Geometry check sheet. Reference: the model listing, model coordinates, mm. A direction names the side the tool comes from. Give positions to 0.01 mm unless a question says otherwise; leave off trailing zeros. Write each loop counter-clockwise with the first axis right and the second up, starting at its lowest first coordinate (ties: lowest second). Pieces come first, ordered by that corner, then holes. Notation, with made-up numbers: M 1.5,14.5 L 5.5,14.5 A23 cw 5.5,43.5 Z; hole C 74,-23 d3. An arc over 180 degrees is marked long. One line per item, written item: value. Start each with the question number.
1. Cross-section at D-D on x = 108.5. Record the cut outline in (y, z).
2. Tool access check on faces 4 (the face through (195.423, -46.748, 39.408)), 5 (the face through (43.2, -23.3, 33.5)), 6 (the face through (196, -47, 37.592)). Record the directions out of +Z, -Z, +X, -X, +Y, -Y that give a thin tool (end or side, any length) a straight path to the whole face; none if there is none.
3. Cross-section at B-B on z = 10. Count the separate pieces of the cut face and the enclosed holes in it, then the cut area to 3 significant figures.
4. Cross-section at C-C on y = -97. Record the cut outline in (x, z) (1 decimal).
5. Gauge pin test, flat ends, axial feed: pin 1 (0.8 mm diameter, centred on y = -98, z = 41, fed in from -X); pin 2 (9.5 mm diameter, centred on x = 62.23, y = -24.13, fed in from -Z); pin 3 (0.8 mm diameter, centred on y = -107.5, z = 41, fed in from +X). Record the tip position at first contact, or that the pin passes through.
6. Release check for a two-part mould opening along Y. For faces 1 (the face through (219.8, -6.44, 19.97)), 2 (the face through (195.423, -110.248, 39.408)), 3 (the face through (111, -74, 0)) record: pulls with the +Y half, pulls with the -Y half, needs draft (parallel to the pull), parting line crosses it, or undercut.
7. Scan lines: line 1 (Y direction, x = 30, z = 19); line 2 (X direction, y = -23, z = 19); line 3 (Y direction, x = 30.48, z = 19.5). Record each from-to range of solid material in increasing order.
8. Cross-section at A-A on x = 163.83. Record the cut outline in (y, z), then the cut area to 3 significant figures.
from build123d import *

# Parameters (mm, degrees)
SKETCH3_W                                        = 226.06
SKETCH3_H                                        = 149.86
EXTRUDE2_DEPTH                                   = 41.275
SKETCH4_W                                        = 226.06
SKETCH4_H                                        = 149.86
SKETCH4_W_2                                      = 22.225
SKETCH4_H_2                                      = 50.8
EXTRUDE4_DEPTH                                   = 0.762
CBORE_FOR_1_4_SOCKET_HEAD_CAP_SCREW1_AT_COUNT    = 2
CBORE_FOR_1_4_SOCKET_HEAD_CAP_SCREW1_AT_PITCH    = 186.028991356
CBORE_FOR_1_4_SOCKET_HEAD_CAP_SCREW1_2_COUNT     = 2
CBORE_FOR_1_4_SOCKET_HEAD_CAP_SCREW1_2_PITCH     = 166.589197204
CBORE_FOR_1_4_SOCKET_HEAD_CAP_SCREW1_3_COUNT     = 2
CBORE_FOR_1_4_SOCKET_HEAD_CAP_SCREW1_3_PITCH     = 63.5
F_1_4_20_TAPPED_HOLE1_D                          = 5.1054
CBORE_FOR_3_8_SOCKET_HEAD_CAP_SCREW1_D           = 10.31748
CBORE_FOR_3_8_SOCKET_HEAD_CAP_SCREW1_CBORE_D     = 38.1
CBORE_FOR_3_8_SOCKET_HEAD_CAP_SCREW1_CBORE_DEPTH = 14.224
SKETCH18_W                                       = 3.175
SKETCH18_H                                       = 133.35
CUT_EXTRUDE1_DEPTH                               = 0.762
F_10_32_TAPPED_HOLE1_D                           = 4.0386
CHAMFER1_SIZE                                    = 12.7


with BuildPart() as part:
    # Sketch3 → Extrude2 (new body)
    with BuildSketch(Plane.XY):
        with Locations((113.03, -74.93)):
            Rectangle(SKETCH3_W, SKETCH3_H)
    extrude(amount=EXTRUDE2_DEPTH)

    # Sketch4 → Extrude4 (cut)
    with BuildSketch(Plane.XY.offset(41.275)):
        with Locations((113.03, -74.93)):
            Rectangle(SKETCH4_W, SKETCH4_H)
        with Locations((30.4927, -33.655)):
            Rectangle(SKETCH4_W_2, SKETCH4_H_2, mode=Mode.SUBTRACT)
        with Locations((195.5673, -33.655)):
            Rectangle(SKETCH4_W_2, SKETCH4_H_2, mode=Mode.SUBTRACT)
        with Locations((30.4927, -116.205)):
            Rectangle(SKETCH4_W_2, SKETCH4_H_2, mode=Mode.SUBTRACT)
        with Locations((195.5673, -116.205)):
            Rectangle(SKETCH4_W_2, SKETCH4_H_2, mode=Mode.SUBTRACT)
    extrude(amount=-EXTRUDE4_DEPTH, mode=Mode.SUBTRACT)

    # Sketch9 → CBORE for 1/4 Socket Head Cap Screw1 (revolve, cut)
    with BuildSketch(Plane(origin=(195.58, -106.68, 0), x_dir=(0, 1, 0), z_dir=(1, 0, 0))):
        Polygon((0, 0), (0, 41.275), (3.57124, 41.275), (3.57124, 37.592), (5.55625, 37.592), (5.55625, 0.635), (6.19125, 0), align=None)
    cbore_for_1_4_socket_head_cap_screw1 = revolve(axis=Axis((195.58, -106.68, -6.35), (0, 0, 1)), mode=Mode.SUBTRACT)

    # CBORE for 1/4 Socket Head Cap Screw1 at: CBORE for 1/4 Socket Head Cap Screw1 ×2
    with Locations(*[Vector(-0.887496077, 0.460815271, 0) * (i * CBORE_FOR_1_4_SOCKET_HEAD_CAP_SCREW1_AT_PITCH) for i in range(1, CBORE_FOR_1_4_SOCKET_HEAD_CAP_SCREW1_AT_COUNT)]):
        add(cbore_for_1_4_socket_head_cap_screw1, mode=Mode.SUBTRACT)

    # CBORE for 1_4 Socket Head Cap Screw1 2: CBORE for 1/4 Socket Head Cap Screw1 ×2
    with Locations(*[Vector(-0.991060662, -0.133412012, 0) * (i * CBORE_FOR_1_4_SOCKET_HEAD_CAP_SCREW1_2_PITCH) for i in range(1, CBORE_FOR_1_4_SOCKET_HEAD_CAP_SCREW1_2_COUNT)]):
        add(cbore_for_1_4_socket_head_cap_screw1, mode=Mode.SUBTRACT)

    # CBORE for 1_4 Socket Head Cap Screw1 3: CBORE for 1/4 Socket Head Cap Screw1 ×2
    with Locations(*[(0, i * CBORE_FOR_1_4_SOCKET_HEAD_CAP_SCREW1_3_PITCH, 0) for i in range(1, CBORE_FOR_1_4_SOCKET_HEAD_CAP_SCREW1_3_COUNT)]):
        add(cbore_for_1_4_socket_head_cap_screw1, mode=Mode.SUBTRACT)

    # 1/4-20 Tapped Hole1 (through all)
    with Locations(Plane(origin=(0, 0, 0), x_dir=(-1, 0, 0), z_dir=(0, 0, -1))):
        with Locations((-195.58, -20.955), (-195.58, -128.905), (-30.48, -43.18), (-30.48, -106.68)):
            Hole(F_1_4_20_TAPPED_HOLE1_D / 2)

    # CBORE for 3/8 Socket Head Cap Screw1 (through all)
    with Locations(Plane.XY.offset(40.513)):
        with Locations((163.83, -125.73), (62.23, -125.73), (163.83, -24.13), (62.23, -24.13)):
            CounterBoreHole(CBORE_FOR_3_8_SOCKET_HEAD_CAP_SCREW1_D / 2, CBORE_FOR_3_8_SOCKET_HEAD_CAP_SCREW1_CBORE_D / 2, CBORE_FOR_3_8_SOCKET_HEAD_CAP_SCREW1_CBORE_DEPTH)

    # Sketch18 → Cut-Extrude1 (cut)
    with BuildSketch(Plane.XY.offset(41.275)):
        with Locations((30.48, -74.93)):
            Rectangle(SKETCH18_W, SKETCH18_H)
        with Locations((195.58, -74.93)):
            Rectangle(SKETCH18_W, SKETCH18_H)
    extrude(amount=-CUT_EXTRUDE1_DEPTH, mode=Mode.SUBTRACT)

    # #10-32 Tapped Hole1 (through all)
    with Locations(Plane(origin=(0, 0, 0), x_dir=(-1, 0, 0), z_dir=(0, 0, -1))):
        with Locations((-113.03, -13.0048), (-100.33, -136.8552), (-125.73, -136.8552)):
            Hole(F_10_32_TAPPED_HOLE1_D / 2)

    # Chamfer1
    chamfer1_edges = [part.edges().sort_by_distance(p)[0] for p in [
        (0, 0, 20.2565),
        (226.06, 0, 20.2565),
        (226.06, -149.86, 20.2565),
        (0, -149.86, 20.2565),
    ]]
    chamfer(chamfer1_edges, length=CHAMFER1_SIZE)


solid = part.part
Report:
1. outline: M -149.86,0 L 0,0 L 0,40.51 L -149.86,40.51 Z
2. face 4: +Z, -Z
2. face 5: +Z
2. face 6: -Z
3. separate pieces: 1
3. enclosed holes: 15
3. area: 32,700 mm^2
4. outline: M 0,0 L 226.1,0 L 226.1,40.5 L 206.7,40.5 L 206.7,41.3 L 197.2,41.3 L 197.2,40.5 L 194,40.5 L 194,41.3 L 184.5,41.3 L 184.5,40.5 L 41.6,40.5 L 41.6,41.3 L 32.1,41.3 L 32.1,40.5 L 28.9,40.5 L 28.9,41.3 L 19.4,41.3 L 19.4,40.5 L 0,40.5 Z
5. pin 1: stops at x = 19.38
5. pin 2: passes through
5. pin 3: stops at x = 206.68
6. face 1: pulls with the +Y half
6. face 2: undercut
6. face 3: needs draft
7. line 1: y = -149.86 to -134.44, -123.37 to -109.19, -104.17 to -45.69, -40.67 to -26.49, -15.42 to 0
7. line 2: x = 0 to 25.31, 35.65 to 57.2, 67.26 to 158.8, 168.86 to 194.05, 197.11 to 226.06
7. line 3: y = -149.86 to -134.46, -123.35 to -109.23, -104.13 to -45.73, -40.63 to -26.51, -15.4 to 0
8. outline: M -149.86,0 L -130.89,0 L -130.89,26.29 L -144.78,26.29 L -144.78,40.51 L -149.86,40.51 Z; M -120.57,0 L -29.29,0 L -29.29,26.29 L -43.18,26.29 L -43.18,40.51 L -106.68,40.51 L -106.68,26.29 L -120.57,26.29 Z; M -18.97,0 L 0,0 L 0,40.51 L -5.08,40.51 L -5.08,26.29 L -18.97,26.29 Z
8. area: 4,440 mm^2
